Source: CAD feature listing. Evaluate the final solid. Frame: model axes, mm. Face numbers are marked on the shaded views. Coordinates: 2 decimals unless noted, no trailing zeros. Order: outer loops, then holes, each group sorted by start corner. A loop starts at its lowest first (then second) coordinate and runs counter-clockwise, first axis right, second up. Notation, with made-up numbers: (8, -14) -> (49, -14) arc R17 ccw to (49, -3) -> close; hole circle Ø7 at (24.5, -28). An arc over 180 degrees is marked (long way). Put each result on its own line as item: value.
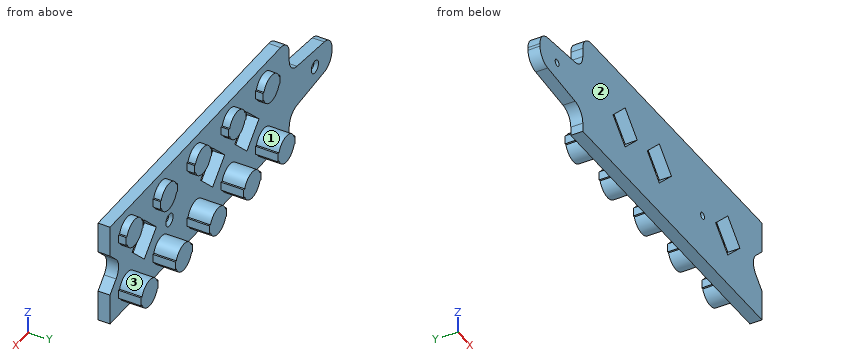
from build123d import *

# Parameters (mm, degrees)
SKETCH1_W           = 259.5
SKETCH1_H           = 70
SKETCH1_R           = 2.25
BOSS_EXTRUDE1_DEPTH = 8
BOSS_EXTRUDE2_DEPTH = 5
BOSS_EXTRUDE3_DEPTH = 15
CHAMFER2_SIZE       = 2
CUT_EXTRUDE2_DEPTH  = 194.184497308
FILLET1_R           = 10


with BuildPart() as part:
    # Sketch1 → Boss-Extrude1 (new body)
    with BuildSketch(Plane(origin=(0, 0, 0), x_dir=(1, 0, 0), z_dir=(0, 1, 0))):
        with Locations((24.75, 80)):
            Rectangle(SKETCH1_W, SKETCH1_H)
        with Locations(Location((-85, 85, 0), (0, 0, 270))):
            Circle(SKETCH1_R, mode=Mode.SUBTRACT)
        with Locations(Location((85, 85, 0), (0, 0, 270))):
            Circle(SKETCH1_R, mode=Mode.SUBTRACT)
    extrude(amount=BOSS_EXTRUDE1_DEPTH)

    # Sketch3 → Boss-Extrude2 (add)
    with BuildSketch(Plane(origin=(0, 8, 0), x_dir=(1, 0, 0), z_dir=(0, 1, 0))):
        with BuildLine():
            Line((-15.5, 57.125), (-15.5, 62.875))
            Line((-15.5, 62.875), (-16.655545523, 62.875))
            ThreePointArc((-16.655545523, 62.875), (-25.5, 69.3), (-34.344454477, 62.875))
            Line((-34.344454477, 62.875), (-35.5, 62.875))
            Line((-35.5, 62.875), (-35.5, 57.125))
            Line((-35.5, 57.125), (-34.344454477, 57.125))
            ThreePointArc((-34.344454477, 57.125), (-25.5, 50.7), (-16.655545523, 57.125))
            Line((-16.655545523, 57.125), (-15.5, 57.125))
        make_face()
        with BuildLine():
            Line((24.5, 57.125), (24.5, 62.875))
            Line((24.5, 62.875), (23.344454477, 62.875))
            ThreePointArc((23.344454477, 62.875), (14.5, 69.3), (5.655545523, 62.875))
            Line((5.655545523, 62.875), (4.5, 62.875))
            Line((4.5, 62.875), (4.5, 57.125))
            Line((4.5, 57.125), (5.655545523, 57.125))
            ThreePointArc((5.655545523, 57.125), (14.5, 50.7), (23.344454477, 57.125))
            Line((23.344454477, 57.125), (24.5, 57.125))
        make_face()
        with BuildLine():
            Line((64.5, 57.125), (64.5, 62.875))
            Line((64.5, 62.875), (63.344454477, 62.875))
            ThreePointArc((63.344454477, 62.875), (54.5, 69.3), (45.655545523, 62.875))
            Line((45.655545523, 62.875), (44.5, 62.875))
            Line((44.5, 62.875), (44.5, 57.125))
            Line((44.5, 57.125), (45.655545523, 57.125))
            ThreePointArc((45.655545523, 57.125), (54.5, 50.7), (63.344454477, 57.125))
            Line((63.344454477, 57.125), (64.5, 57.125))
        make_face()
        with BuildLine():
            Line((104.5, 57.125), (104.5, 62.875))
            Line((104.5, 62.875), (103.344454477, 62.875))
            ThreePointArc((103.344454477, 62.875), (94.5, 69.3), (85.655545523, 62.875))
            Line((85.655545523, 62.875), (84.5, 62.875))
            Line((84.5, 62.875), (84.5, 57.125))
            Line((84.5, 57.125), (85.655545523, 57.125))
            ThreePointArc((85.655545523, 57.125), (94.5, 50.7), (103.344454477, 57.125))
            Line((103.344454477, 57.125), (104.5, 57.125))
        make_face()
        with BuildLine():
            Line((144.5, 57.125), (144.5, 62.875))
            Line((144.5, 62.875), (143.344454477, 62.875))
            ThreePointArc((143.344454477, 62.875), (134.5, 69.3), (125.655545523, 62.875))
            Line((125.655545523, 62.875), (124.5, 62.875))
            Line((124.5, 62.875), (124.5, 57.125))
            Line((124.5, 57.125), (125.655545523, 57.125))
            ThreePointArc((125.655545523, 57.125), (134.5, 50.7), (143.344454477, 57.125))
            Line((143.344454477, 57.125), (144.5, 57.125))
        make_face()
    extrude(amount=BOSS_EXTRUDE2_DEPTH)

    # Sketch3<3> → Boss-Extrude3 (add)
    with BuildSketch(Plane(origin=(0, 8, 0), x_dir=(1, 0, 0), z_dir=(0, 1, 0))):
        with BuildLine():
            Line((24.5, 97.125), (24.5, 102.875))
            Line((24.5, 102.875), (23.344454477, 102.875))
            ThreePointArc((23.344454477, 102.875), (14.5, 109.3), (5.655545523, 102.875))
            Line((5.655545523, 102.875), (4.5, 102.875))
            Line((4.5, 102.875), (4.5, 97.125))
            Line((4.5, 97.125), (5.655545523, 97.125))
            ThreePointArc((5.655545523, 97.125), (14.5, 90.7), (23.344454477, 97.125))
            Line((23.344454477, 97.125), (24.5, 97.125))
        make_face()
        with BuildLine():
            Line((64.5, 97.125), (64.5, 102.875))
            Line((64.5, 102.875), (63.344454477, 102.875))
            ThreePointArc((63.344454477, 102.875), (54.5, 109.3), (45.655545523, 102.875))
            Line((45.655545523, 102.875), (44.5, 102.875))
            Line((44.5, 102.875), (44.5, 97.125))
            Line((44.5, 97.125), (45.655545523, 97.125))
            ThreePointArc((45.655545523, 97.125), (54.5, 90.7), (63.344454477, 97.125))
            Line((63.344454477, 97.125), (64.5, 97.125))
        make_face()
        with BuildLine():
            Line((104.5, 97.125), (104.5, 102.875))
            Line((104.5, 102.875), (103.344454477, 102.875))
            ThreePointArc((103.344454477, 102.875), (94.5, 109.3), (85.655545523, 102.875))
            Line((85.655545523, 102.875), (84.5, 102.875))
            Line((84.5, 102.875), (84.5, 97.125))
            Line((84.5, 97.125), (85.655545523, 97.125))
            ThreePointArc((85.655545523, 97.125), (94.5, 90.7), (103.344454477, 97.125))
            Line((103.344454477, 97.125), (104.5, 97.125))
        make_face()
        with BuildLine():
            Line((144.5, 97.125), (144.5, 102.875))
            Line((144.5, 102.875), (143.344454477, 102.875))
            ThreePointArc((143.344454477, 102.875), (134.5, 109.3), (125.655545523, 102.875))
            Line((125.655545523, 102.875), (124.5, 102.875))
            Line((124.5, 102.875), (124.5, 97.125))
            Line((124.5, 97.125), (125.655545523, 97.125))
            ThreePointArc((125.655545523, 97.125), (134.5, 90.7), (143.344454477, 97.125))
            Line((143.344454477, 97.125), (144.5, 97.125))
        make_face()
        with BuildLine():
            Line((-15.5, 97.125), (-15.5, 102.875))
            Line((-15.5, 102.875), (-16.655545523, 102.875))
            ThreePointArc((-16.655545523, 102.875), (-25.5, 109.3), (-34.344454477, 102.875))
            Line((-34.344454477, 102.875), (-35.5, 102.875))
            Line((-35.5, 102.875), (-35.5, 97.125))
            Line((-35.5, 97.125), (-34.344454477, 97.125))
            ThreePointArc((-34.344454477, 97.125), (-25.5, 90.7), (-16.655545523, 97.125))
            Line((-16.655545523, 97.125), (-15.5, 97.125))
        make_face()
    extrude(amount=BOSS_EXTRUDE3_DEPTH)

    # Chamfer2
    chamfer2_edges = [part.edges().sort_by_distance(p)[0] for p in [
        (-85, 8, -87.25),
        (85, 8, -87.25),
    ]]
    chamfer(chamfer2_edges, length=CHAMFER2_SIZE)

    # Sketch5 → Cut-Extrude2 (cut, through all)
    with BuildSketch(Plane(origin=(0, 8, 0), x_dir=(1, 0, 0), z_dir=(0, 1, 0))):
        Polygon((-55, 70), (-105, 75), (-105, 45), (-55, 45), align=None)
        Polygon((34.5, 65.857864376), (48.642135624, 80), (34.5, 94.142135624), (20.357864376, 80), align=None)
        Polygon((-105, 115), (-105, 95), (-55, 100), (-55, 115), align=None)
        Polygon((114.5, 65.857864376), (128.642135624, 80), (114.5, 94.142135624), (100.357864376, 80), align=None)
        Polygon((154.5, 65.857864376), (168.642135624, 80), (154.5, 94.142135624), (140.357864376, 80), align=None)
        Polygon((-5.5, 65.857864376), (8.642135624, 80), (-5.5, 94.142135624), (-19.642135624, 80), align=None)
    extrude(amount=-CUT_EXTRUDE2_DEPTH, mode=Mode.SUBTRACT)

    # Fillet1
    fillet1_edges = [part.edges().sort_by_distance(p)[0] for p in [
        (140.357864376, 4, -80),
        (-55, 4, -100),
        (-105, 4, -95),
        (-105, 4, -75),
        (-55, 4, -70),
        (-55, 4, -45),
    ]]
    fillet(fillet1_edges, radius=FILLET1_R)


solid = part.part
1. Cut plane A-A on x = -85. Output: boundary loops of the cut face in (y, z), plus the area to 3 significant figures.
Numbers:
outline: (0, -97) -> (8, -97) -> (8, -89.25) -> (6, -87.25) -> (0, -87.25) -> close; (0, -82.75) -> (6, -82.75) -> (8, -80.75) -> (8, -73) -> (0, -73) -> close
area: 152 mm2
2. First-contact query: pin 1 (0.6 mm diameter, centred on x = 125, y = 10.5, fed in from +Z) (3 decimals); pin 2 (3 mm diameter, centred on x = 6.5, z = -65.5, fed in from +Y); pin 3 (8 mm diameter, centred on y = 10.5, z = -66, fed in from -X); pin 4 (4 mm diameter, centred on x = -36, y = 9.5, fed in from +Z). Flat tips, straight axial feed; report the tip coordinate or a pass-through.
Numbers:
pin 1: stops at z = -57.125
pin 2: stops at y = 13
pin 3: stops at x = -59.24
pin 4: stops at z = -45
3. Ray query, line 1 along X through (y, z) = (4.75, -77.5); line 2 along X through (y, z) = (3.5, -76); line 3 along X through (y, z) = (18.5, -97). Return the intervals inside material, ascending.
Numbers:
line 1: x = -102.56 to -17.14, 6.14 to 22.86, 46.14 to 102.86, 126.14 to 144.82
line 2: x = -100.93 to -15.64, 4.64 to 24.36, 44.64 to 104.36, 124.64 to 145.33
line 3: x = -34.3 to -16.7, 5.7 to 23.3, 45.7 to 63.3, 85.7 to 103.3, 125.7 to 143.3
4. Pull-direction query (X, two-part tool) for the marked faces 1, 2 and 3; classes: pulls with the +X half, pulls with the -X half, needs draft (parallel to the pull), parting line crosses it, or undercut.
Numbers:
face 1: undercut
face 2: needs draft
face 3: undercut
5. Cut plane D-D on x = -27. Output: boundary loops of the cut face in (y, z).
Numbers:
outline: (0, -115) -> (8, -115) -> (8, -109.18) -> (23, -109.18) -> (23, -90.82) -> (8, -90.82) -> (8, -69.18) -> (13, -69.18) -> (13, -50.82) -> (8, -50.82) -> (8, -45) -> (0, -45) -> close
6. Cut plane C-C on x = 112. Output: boundary loops of the cut face in (y, z), plus the area to 3 significant figures.
Numbers:
outline: (0, -115) -> (8, -115) -> (8, -91.64) -> (0, -91.64) -> close; (0, -68.36) -> (8, -68.36) -> (8, -45) -> (0, -45) -> close
area: 374 mm2
7. Cut plane B-B on y = 17. Count the separate pieces of the cut face and the enclosed holes in it, plus the area to 3 significant figures.
Numbers:
separate pieces: 5
enclosed holes: 0
area: 1,410 mm2
